from build123d import *

# Parameters (mm, degrees)
F1_DEPTH = 30
F2_R     = 7.5
F2_R_2   = 6
F3_DEPTH = 13.001


with BuildPart() as f1:
    # F0 (on Front) → F1 (new body)
    with BuildSketch(Plane.XZ):
        Polygon((62, 0), (0, 0), (0, -13), (10, -13), (10, -3), (52, -3), (52, -13), (62, -13), align=None)
    extrude(amount=F1_DEPTH)

    # F2 (on face) → F3 (cut, through all)
    with BuildSketch(Plane.XY):
        with Locations((20, -15)):
            Circle(F2_R)
        with Locations((42, -15)):
            Circle(F2_R_2)
    extrude(amount=-F3_DEPTH, mode=Mode.SUBTRACT)


solid = f1.part
Source: CAD feature listing. Evaluate the final solid. Frame: model axes, mm. A direction names the side the tool comes from. Coordinates: 2 decimals unless noted, no trailing zeros. Loops run counter-clockwise (first coordinate to the right, second up) from the corner with the lowest first, then second, coordinate; pieces in that order, holes last. Notation, with made-up numbers: M 40,-17 L 54,-17 A24 cw 54,19 Z; hole C -10,64 d1. An arc over 180 degrees is marked long. Answer in a Markdown table with one row per item.
Q1. Section C-C on x = 42. Return the cut outline in (y, z), plus the area to 3 significant figures.
Answers below:
| item | result |
|---|---|
| outline | M -30,-3 L -21,-3 L -21,0 L -30,0 Z; M -9,-3 L 0,-3 L 0,0 L -9,0 Z |
| area | 54.0 mm^2 |
Q2. Section D-D on z = -2.25. Return the cut outline in (x, y), plus the area to 3 significant figures.
Answers below:
| item | result |
|---|---|
| outline | M 0,-30 L 62,-30 L 62,0 L 0,0 Z; hole C 20,-15 d15; hole C 42,-15 d12 |
| area | 1,570 mm^2 |
Q3. Section B-B on y = -15. Return the cut outline in (x, z).
Answers below:
| item | result |
|---|---|
| outline | M 0,-13 L 10,-13 L 10,-3 L 12.5,-3 L 12.5,0 L 0,0 Z; M 27.5,-3 L 36,-3 L 36,0 L 27.5,0 Z; M 48,-3 L 52,-3 L 52,-13 L 62,-13 L 62,0 L 48,0 Z |
Q4. Set-up query: faces 1 (the flat face through (10, -15, -8)), 2 (the flat face through (31, -15, 0)). Return all of +Z, -Z, +X, -X, +Y, -Y with unobstructed straight access to the full face (end or side cutting, diameter ignored); none if empty.
Answers below:
| item | result |
|---|---|
| face 1 | -Z, +Y, -Y |
| face 2 | +Z, +X, -X, +Y, -Y |
Q5. Ray query, probe 1 along X at (y, z) = (-4.5, -3.75); probe 2 along Y at (x, z) = (20, -0.9); probe 3 along Y at (x, z) = (42, -1.3). Return the intervals inside material, ascending. Write a range as from..to.
Answers below:
| item | result |
|---|---|
| probe 1 | x = 0..10, 52..62 |
| probe 2 | y = -30..-22.5, -7.5..0 |
| probe 3 | y = -30..-21, -9..0 |
Q6. First-contact query: pin 1 (9 mm diameter, centred on x = 22, y = -12.5, fed in from -Z). Flat tip, straight axial feed; report the tip coordinate or a pass-through.
Answers below:
| item | result |
|---|---|
| pin 1 | stops at z = -3 |
Q7. Section A-A on z = -10.5. Return the cut outline in (x, y).
Answers below:
| item | result |
|---|---|
| outline | M 0,-30 L 10,-30 L 10,0 L 0,0 Z; M 52,-30 L 62,-30 L 62,0 L 52,0 Z |
Q8. Draft query along X for faces 3 (the flat face through (31, -15, -3)), 4 (the flat face through (57, -15, -13)), 5 (the flat face through (62, -15, -7)). Return one class per face: pulls with the +X half, pulls with the -X half, needs draft (parallel to the pull), parting line crosses it, or undercut.
Answers below:
| item | result |
|---|---|
| face 3 | undercut |
| face 4 | needs draft |
| face 5 | pulls with the +X half |
